Input: part model. Units: mm. Frame: model coordinates. Face numbers are marked on the shaded views. A direction names the side the tool comes from. Give positions to 0.01 mm unless a question says otherwise; leave off trailing zeros. Loops run counter-clockwise (first coordinate to the right, second up) from the corner with the lowest first, then second, coordinate; pieces in that order, holes last. Notation, with made-up numbers: (57, -36) - (114, -36) arc R11 cw to (114, -18) - close; hole circle Ø11 at (30.25, 44). An arc over 180 degrees is marked (long way). One line per item, written item: value.
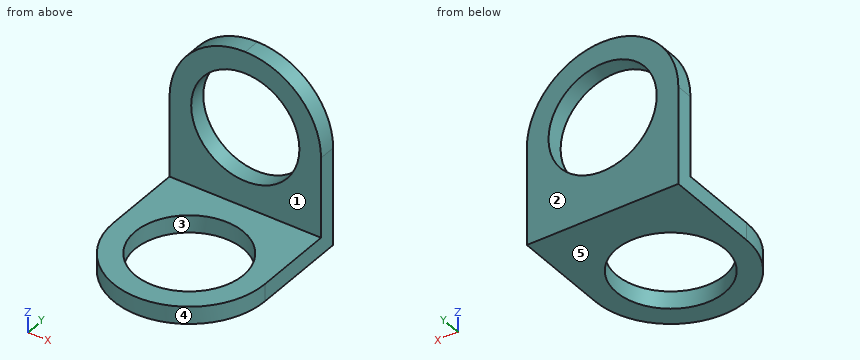
from build123d import *

# Parameters (mm, degrees)
F0_R     = 12.5
F1_DEPTH = 4
F2_W     = 35
F2_H     = 4
F3_DEPTH = 36
F4_R     = 12.5
F5_DEPTH = 25


with BuildPart() as f1:
    # F0 (on Top) → F1 (new body)
    with BuildSketch(Plane.XY):
        with BuildLine():
            Line((17.5, 0.575275), (-17.5, 0.575275))
            Line((-17.5, 0.575275), (-17.5, -21.924725))
            ThreePointArc((-17.5, -21.924725), (0, -39.424725), (17.5, -21.924725))
            Line((17.5, -21.924725), (17.5, 0.575275))
        make_face()
        with Locations((0, -21.924725)):
            Circle(F0_R, mode=Mode.SUBTRACT)
    extrude(amount=F1_DEPTH)

    # F2 (on face) → F3 (join)
    with BuildSketch(Plane.XY.offset(4)):
        with Locations((0, -1.424725)):
            Rectangle(F2_W, F2_H)
    extrude(amount=F3_DEPTH)

    # F4 (on face) → F5 (cut)
    with BuildSketch(Plane.XZ.offset(3.424725)):
        with BuildLine():
            ThreePointArc((-17.5, 22.5), (-12.374369, 34.874369), (0, 40))
            Line((0, 40), (-17.5, 40))
            Line((-17.5, 40), (-17.5, 22.5))
        make_face()
        with BuildLine():
            ThreePointArc((0, 40), (12.374369, 34.874369), (17.5, 22.5))
            Line((17.5, 22.5), (17.5, 40))
            Line((17.5, 40), (0, 40))
        make_face()
        with Locations((0, 22.5)):
            Circle(F4_R)
    extrude(amount=-F5_DEPTH, mode=Mode.SUBTRACT)


solid = f1.part
Item 1: Access query for the marked faces 1 and 2. Directions: +Z, -Z, +X, -X, +Y, -Y. A direction counts if a zero-diameter tool reaches every point of the face in a straight line with its end or side. Return the directions, or none.
Verdict:
face 1: +Z, +X, -X, -Y
face 2: +Z, -Z, +X, -X, +Y
Item 2: Section B-B, the plane z = 21. Output: boundary loops of the cut face in (x, y).
Verdict:
outline: (-17.5, -3.42) - (-12.41, -3.42) - (-12.41, 0.58) - (-17.5, 0.58) - close; (12.41, -3.42) - (17.5, -3.42) - (17.5, 0.58) - (12.41, 0.58) - close
Item 3: Draft query along X for the marked faces 3, 4 and 5. Return one class per face: pulls with the +X half, pulls with the -X half, needs draft (parallel to the pull), parting line crosses it, or undercut.
Verdict:
face 3: undercut
face 4: parting line crosses it
face 5: needs draft
Item 4: Section A-A, the plane y = -17. Output: boundary loops of the cut face in (x, z), and give its area (3 significant figures).
Verdict:
outline: (-17.5, 0) - (-11.49, 0) - (-11.49, 4) - (-17.5, 4) - close; (11.49, 0) - (17.5, 0) - (17.5, 4) - (11.49, 4) - close
area: 48.1 mm^2
Item 5: Section C-C, the plane x = -10. Output: boundary loops of the cut face in (y, z), and give its area (3 significant figures).
Verdict:
outline: (-36.29, 0) - (-29.42, 0) - (-29.42, 4) - (-36.29, 4) - close; (-14.42, 0) - (0.58, 0) - (0.58, 15) - (-3.42, 15) - (-3.42, 4) - (-14.42, 4) - close; (-3.42, 30) - (0.58, 30) - (0.58, 36.86) - (-3.42, 36.86) - close
area: 159 mm^2
Item 6: Section D-D, the plane x = -15. Output: boundary loops of the cut face in (y, z), and give its area (3 significant figures).
Verdict:
outline: (-30.94, 0) - (0.58, 0) - (0.58, 31.51) - (-3.42, 31.51) - (-3.42, 4) - (-30.94, 4) - close
area: 236 mm^2
Item 7: Pin query (flat end, axial travel): P1, Ø1.5, axis at x = 9.5, z = 33.5, coming from the -Y side. Return the tip coordinate at first contact, or that it passes through.
Verdict:
P1: stops at y = -3.42
Item 8: Material intervals for L1, parallel to Z at x = 0, y = -2; L2, parallel to Z at x = 13, y = -22; L3, parallel to X at y = -2, z = 28.5, sorted ascending.
Verdict:
L1: z = 0 to 10, 35 to 40
L2: z = 0 to 4
L3: x = -16.44 to -10.97, 10.97 to 16.44
